from build123d import *

# Parameters (mm, degrees)
F1_DEPTH = 150
F3_DEPTH = 25


with BuildPart() as f1:
    # F0 (on Right) → F1 (new body)
    with BuildSketch(Plane.YZ):
        with BuildLine():
            ThreePointArc((0, 39), (0.292893, 39.707107), (1, 40))
            Line((1, 40), (18.8, 40))
            ThreePointArc((18.8, 40), (19.507107, 39.707107), (19.8, 39))
            Line((19.8, 39), (19.8, 2))
            ThreePointArc((19.8, 2), (20.385786, 0.585786), (21.8, 0))
            ThreePointArc((21.8, 0), (23.214214, 0.585786), (23.8, 2))
            Line((23.8, 2), (23.8, 41.485587))
            ThreePointArc((23.8, 41.485587), (24.815656, 44.506349), (27.45, 46.299889))
            ThreePointArc((27.45, 46.299889), (35.675412, 49.791064), (42.748737, 55.251263))
            Line((42.748737, 55.251263), (47.698485, 60.20101))
            ThreePointArc((47.698485, 60.20101), (47.991378, 60.908117), (47.698485, 61.615224))
            Line((47.698485, 61.615224), (46.991378, 62.32233))
            ThreePointArc((46.991378, 62.32233), (46.284271, 62.615224), (45.577164, 62.32233))
            Line((45.577164, 62.32233), (40.627417, 57.372583))
            ThreePointArc((40.627417, 57.372583), (-4.28194, 57.032302), (-5.302705, 101.931346))
            ThreePointArc((-5.302705, 101.931346), (-5.031029, 102.631854), (-5.323808, 103.323808))
            Line((-5.323808, 103.323808), (-6.03123, 104.03123))
            ThreePointArc((-6.03123, 104.03123), (-6.753044, 104.324015), (-7.465935, 104.010127))
            ThreePointArc((-7.465935, 104.010127), (-16.976143, 78.707928), (-5.625, 54.17638))
            ThreePointArc((-5.625, 54.17638), (-4.424249, 52.502855), (-4, 50.487291))
            Line((-4, 50.487291), (-4, 2))
            ThreePointArc((-4, 2), (-3.414214, 0.585786), (-2, 0))
            ThreePointArc((-2, 0), (-0.585786, 0.585786), (0, 2))
            Line((0, 2), (0, 39))
        make_face()
    extrude(amount=F1_DEPTH)

    # F2 (on Front) → F3 (cut)
    with BuildSketch(Plane.XZ):
        with BuildLine():
            Line((14, 114.010127), (10, 114.010127))
            Line((10, 114.010127), (10, 81.010127))
            ThreePointArc((10, 81.010127), (10.585786, 79.595913), (12, 79.010127))
            ThreePointArc((12, 79.010127), (13.414214, 79.595913), (14, 81.010127))
            Line((14, 81.010127), (14, 114.010127))
        make_face()
        with BuildLine():
            Line((32, 81.010127), (32, 114.010127))
            Line((32, 114.010127), (28, 114.010127))
            Line((28, 114.010127), (28, 81.010127))
            ThreePointArc((28, 81.010127), (28.585786, 79.595913), (30, 79.010127))
            ThreePointArc((30, 79.010127), (31.414214, 79.595913), (32, 81.010127))
        make_face()
        with BuildLine():
            Line((50, 81.010127), (50, 114.010127))
            Line((50, 114.010127), (46, 114.010127))
            Line((46, 114.010127), (46, 81.010127))
            ThreePointArc((46, 81.010127), (46.585786, 79.595913), (48, 79.010127))
            ThreePointArc((48, 79.010127), (49.414214, 79.595913), (50, 81.010127))
        make_face()
        with BuildLine():
            Line((68, 81.010127), (68, 114.010127))
            Line((68, 114.010127), (64, 114.010127))
            Line((64, 114.010127), (64, 81.010127))
            ThreePointArc((64, 81.010127), (64.585786, 79.595913), (66, 79.010127))
            ThreePointArc((66, 79.010127), (67.414214, 79.595913), (68, 81.010127))
        make_face()
        with BuildLine():
            Line((86, 81.010127), (86, 114.010127))
            Line((86, 114.010127), (82, 114.010127))
            Line((82, 114.010127), (82, 81.010127))
            ThreePointArc((82, 81.010127), (82.585786, 79.595913), (84, 79.010127))
            ThreePointArc((84, 79.010127), (85.414214, 79.595913), (86, 81.010127))
        make_face()
        with BuildLine():
            Line((104, 81.010127), (104, 114.010127))
            Line((104, 114.010127), (100, 114.010127))
            Line((100, 114.010127), (100, 81.010127))
            ThreePointArc((100, 81.010127), (100.585786, 79.595913), (102, 79.010127))
            ThreePointArc((102, 79.010127), (103.414214, 79.595913), (104, 81.010127))
        make_face()
        with BuildLine():
            Line((122, 81.010127), (122, 114.010127))
            Line((122, 114.010127), (118, 114.010127))
            Line((118, 114.010127), (118, 81.010127))
            ThreePointArc((118, 81.010127), (118.585786, 79.595913), (120, 79.010127))
            ThreePointArc((120, 79.010127), (121.414214, 79.595913), (122, 81.010127))
        make_face()
        with BuildLine():
            Line((140, 81.010127), (140, 114.010127))
            Line((140, 114.010127), (136, 114.010127))
            Line((136, 114.010127), (136, 81.010127))
            ThreePointArc((136, 81.010127), (136.585786, 79.595913), (138, 79.010127))
            ThreePointArc((138, 79.010127), (139.414214, 79.595913), (140, 81.010127))
        make_face()
    extrude(amount=F3_DEPTH, mode=Mode.SUBTRACT)


solid = f1.part
The model under review builds one solid part; all positions refer to its coordinate system, in mm. A direction names the side the tool comes from. Give positions to 0.01 mm unless a question says otherwise; leave off trailing zeros. Write each loop counter-clockwise with the first axis right and the second up, starting at its lowest first coordinate (ties: lowest second). Pieces come first, ordered by that corner, then holes.
1. Add section C-C, the plane y = 33.5. Write out the cut boundary in (x, z).
2. Tool access review of faces 1 (the flat face through (0, 8, 41)), 2 (the flat face through (74, 0, 20)), 3 (the flat face through (28, -12, 93)), 4 (the flat face through (74, 23.8, 21)), 5 (the flat face through (150, 8, 41)): name each direction out of +Z, -Z, +X, -X, +Y, -Y from which nothing blocks a thin tool from reaching the whole face with its end or side.
3. Add section B-B, the plane x = 110.5. Write out the cut boundary in (y, z) (3 decimals).
4. Add section A-A, the plane z = 25.5. Write out the cut boundary in (x, y).
5. Wall thickness on L1, parallel to Y at x = 118, z = 28.5; L2, parallel to Y at x = 125, z = 55; L3, parallel to Y at x = 112.5, z = 72: over which ranges is each line inside the solid? List them lowest first.
6. For P1, Ø5, axis at x = 116.5, y = 34, coming from the -Z side; P2, Ø2, axis at x = 81.5, z = 12, coming from the -Y side; P3, Ø1.5, axis at x = 72.5, z = 14, coming from the +Y side; P4, Ø3.5, axis at y = -9.5, z = 88, coming from the -X side, all flat-tipped, find the tip position at first contact; note any pin that passes through.
7. Draft analysis for pull direction Y (two halves, no side actions). For faces 6 (the flat face through (74, 19.8, 21)), 7 (the cylindrical face through (73.95, -16.99, 79.1)), 8 (the flat face through (82, -12, 93)), state which applies: +Y half, -Y half, draft (parallel to the pull), parting line (faces both ways), or undercut.
Worked answers:
1. outline: (0, 48.62) - (150, 48.62) - (150, 52) - (0, 52) - close
2. face 1: +Z, -Z, -X, +Y, -Y
2. face 2: -Z, +X, -X
2. face 3: +Z, +Y, -Y
2. face 4: -Z, +X, -X, +Y
2. face 5: +Z, -Z, +X, +Y, -Y
3. outline: (-7.466, 104.01) arc R35 ccw to (-5.625, 54.176) arc R5 cw to (-4, 50.487) - (-4, 2) arc R2 ccw to (-2, 0) arc R2 ccw to (0, 2) - (0, 39) arc R1 cw to (1, 40) - (18.8, 40) arc R1 cw to (19.8, 39) - (19.8, 2) arc R2 ccw to (21.8, 0) arc R2 ccw to (23.8, 2) - (23.8, 41.486) arc R5 cw to (27.45, 46.3) arc R35 ccw to (42.749, 55.251) - (47.698, 60.201) arc R1 ccw to (47.698, 61.615) - (46.991, 62.322) arc R1 ccw to (45.577, 62.322) - (40.627, 57.373) arc R32 cw to (-5.303, 101.931) arc R1 ccw to (-5.324, 103.324) - (-6.031, 104.031) arc R1 ccw to start
4. outline: (0, -4) - (150, -4) - (150, 0) - (0, 0) - close; (0, 19.8) - (150, 19.8) - (150, 23.8) - (0, 23.8) - close
5. L1: y = -4 to 0, 19.8 to 23.8
5. L2: y = -6.49 to -1.97, 37.97 to 42.49
5. L3: y = -16.07 to -12.98
6. P1: stops at z = 47.71
6. P2: stops at y = -4
6. P3: stops at y = 23.8
6. P4: passes through
7. face 6: undercut
7. face 7: -Y half
7. face 8: draft
